Here's how the part is built. I have some questions about the finished solid (model axes, mm). A direction names the side the tool comes from. Coordinates: 2 decimals unless noted, no trailing zeros. Write each loop counter-clockwise with the first axis right and the second up, starting at its lowest first coordinate (ties: lowest second). Pieces come first, ordered by that corner, then holes.
Autodesk Inventor part; units mm, degrees
ref_plane "YZ Plane" through (0, 0, 0) normal (1, 0, 0) x (0, 1, 0)
ref_plane "XZ Plane" through (0, 0, 0) normal (0, 1, 0) x (-1, 0, 0)
ref_plane "XY Plane" through (0, 0, 0) normal (0, 0, 1) x (1, 0, 0)
sketch "Sketch1" plane through (0, 0, 0) normal (0, 0, 1) x (1, 0, 0)
  line L0 (0, 0) -> (0, 5)
  line L1 (0, 5) -> (-27, 5)
  line L2 (-27, 5) -> (-27, -31)
  line L3 (-27, -31) -> (-13, -31)
  arc A0 (0, 0) -> (-12.903, -26.393) centre (26.9732, -29.5372) ccw
  arc A1 (-17.8875, -31) -> (-12.903, -26.393) centre (-17.8875, -26) ccw
  dimension "d3" = 5
  dimension "d4" = 27
  dimension "d5" = 36
  dimension "d6" = 14
  dimension "d9" = 40
  dimension "d10" = 10
extrude "Extrusion1" add sketch "Sketch1" along normal blind 2.5
sketch "Sketch4" plane through (-27, 5, 0) normal (0, 1, 0) x (1, 0, 0)
  circle A0 centre (18, -7.5) radius 2
  line L0 (0, 0) -> (0, -2.5)
  line L1 (27, 0) -> (0, 0)
  point P0 (0, -12)
  dimension "d20" = 4
  dimension "d21" = 18
  dimension "d22" = 7.5
hole "Hole1" at (-9, 5, 7.5) direction (0, -1, 0) diameter 4 end through all
sketch "Sketch5" plane through (0, 0, 2.5) normal (0, 0, 1) x (1, 0, 0)
  line L0 (-22.5, -4) -> (-22.5, -26) construction
  circle A0 centre (-22.5, -4) radius 2
  circle A1 centre (-22.5, -15) radius 2
  circle A2 centre (-22.5, -26) radius 2
  line L1 (-27, 5) -> (0, 5)
  line L2 (-27, 5) -> (-27, -31)
  point P0 (0, 0)
  point P1 (-27, 2.5)
  dimension "d30" = 4
  dimension "d31" = 4
  dimension "d32" = 4
  dimension "d33" = 11
  dimension "d34" = 9
  dimension "d35" = 11
  dimension "d36" = 4.5
hole "Hole2" at (-22.5, -4, 2.5) at (-22.5, -15, 2.5) at (-22.5, -26, 2.5) direction (0, 0, -1) diameter 4 end through all
sketch "Sketch6" plane through (-27, 5, 0) normal (0, 1, 0) x (1, 0, 0)
  line L0 (27, -2.5) -> (0, -2.5)
  line L1 (0, -2.5) -> (0, 9.5)
  line L2 (0, 9.5) -> (27, 9.5)
  line L3 (27, 9.5) -> (27, -2.5)
  line L4 (27, -2.5) -> (0, -2.5)
  line L5 (27, 0) -> (0, 0)
  dimension "d44" = 0
  dimension "d45" = 12
  dimension "d46" = 27
extrude "Extrusion3" add sketch "Sketch6" against normal blind 2.5 contours L5 L1 L2 L3
sketch "Sketch7" plane through (-27, 5, 2.5) normal (0, 1, 0) x (1, 0, 0)
  circle A0 centre (18, 7.5) radius 2
  line L0 (27, 0) -> (0, 0)
  line L1 (0, 12) -> (0, 0)
  point P0 (27, 2.5)
  dimension "d49" = 4
  dimension "d50" = 7.5
  dimension "d51" = 18
hole "Hole3" at (-9, 5, -5) direction (0, -1, 0) diameter 4 end through all
properties part number "1-19"
1) Imagine slicing it at B-B on z = -5. Please give me the cut outline in (x, y).
Values follow:
outline: (-27, 2.5) - (-11, 2.5) - (-11, 5) - (-27, 5) - close; (-7, 2.5) - (0, 2.5) - (0, 5) - (-7, 5) - close
2) We'd pull the mould along Y, two halves only. Please class faces 3 (the face through (-14.46, -29.64, 1.23)), 4 (the face through (-17, -10, 0)), 5 (the face through (-21.3, -13.4, 1.2)), 6 (the face through (-21.3, -2.4, 1.2)): pulls with the +Y half, pulls with the -Y half, needs draft (parallel to the pull), parting line crosses it, or undercut.
Values follow:
face 3: pulls with the -Y half
face 4: needs draft
face 5: undercut
face 6: undercut
3) Imagine slicing it at D-D on x = -10.25. Please give me the cut outline in (y, z), then the cut area to 3 significant figures.
Values follow:
outline: (-14.89, 0) - (2.5, 0) - (2.5, -3.44) - (5, -3.44) - (5, 2.5) - (-14.89, 2.5) - close; (2.5, -9.5) - (5, -9.5) - (5, -6.56) - (2.5, -6.56) - close
area: 65.7 mm2
4) Imagine slicing it at C-C on y = -2.5. Please give me the cut outline in (x, z).
Values follow:
outline: (-27, 0) - (-23.82, 0) - (-23.82, 2.5) - (-27, 2.5) - close; (-21.18, 0) - (-2.51, 0) - (-2.51, 2.5) - (-21.18, 2.5) - close
5) Imagine slicing it at A-A on x = -22.5. Please give me the cut outline in (y, z).
Values follow:
outline: (-31, 0) - (-28, 0) - (-28, 2.5) - (-31, 2.5) - close; (-24, 0) - (-17, 0) - (-17, 2.5) - (-24, 2.5) - close; (-13, 0) - (-6, 0) - (-6, 2.5) - (-13, 2.5) - close; (-2, 0) - (2.5, 0) - (2.5, -9.5) - (5, -9.5) - (5, 2.5) - (-2, 2.5) - close
6) On a 3-axis mill with a long thin cutter (end or side, diameter ignored), from which of +Z, -Z, +X, -X, +Y, -Y can I reach the whole of each face in a straight line? I mean faces 1 (the face through (-14, 2.5, -5)), 2 (the face through (-14, 4, -9.5)). Say none if no direction works.
Values follow:
face 1: -Z, +X, -X, -Y
face 2: -Z, +X, -X, +Y, -Y
7) I need wall thicknesses on probe 1 along Y at (x, z) = (-22.5, 1.9); probe 2 along X at (y, z) = (3.3, -5); probe 3 along Z at (x, y) = (-13.25, -17.5). Which ranges of each line are inside material? Lowest first, please.
Values follow:
probe 1: y = -31 to -28, -24 to -17, -13 to -6, -2 to 5
probe 2: x = -27 to -11, -7 to 0
probe 3: z = 0 to 2.5
8) Will these pins go through, and if not, where does the flat tip stop? pin 1 (4.5 mm diameter, centred on x = -9, z = -5, fed in from -Y); pin 2 (8 mm diameter, centred on x = -20, y = -20, fed in from -Z); pin 3 (1 mm diameter, centred on x = -3, z = 0.5, fed in from -Y).
Values follow:
pin 1: stops at y = 2.5
pin 2: stops at z = 0
pin 3: stops at y = -3.63
